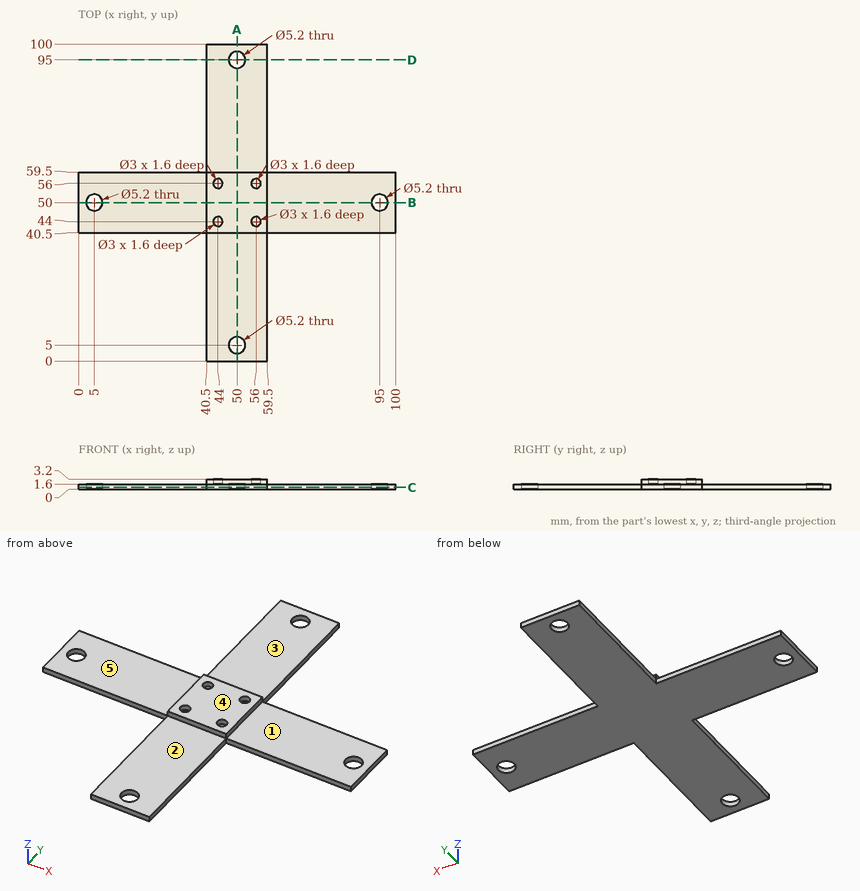
Geometry check sheet. Reference: drawing and pictorial views, mm from the part's lowest x, y, z. A direction names the side the tool comes from. Give positions to 0.01 mm unless a question says otherwise; leave off trailing zeros. Loops run counter-clockwise (first coordinate to the right, second up) from the corner with the lowest first, then second, coordinate; pieces in that order, holes last. Notation, with made-up numbers: (28, 31) -> (65, 31) arc R16 ccw to (65, 46) -> close; hole circle Ø6 at (80.5, 74). An arc over 180 degrees is marked (long way). Answer in a Markdown table with one row per item. Add a question column.
1) Set-up check for the marked faces 1, 2, 3, 4 and 5: record each of +Z, -Z, +X, -X, +Y, -Y from which the full face is reachable in a straight line by a thin tool's end or side.
2) Cross-section at A-A on x = 50. Record the boundary of the cut face in (y, z).
3) Cross-section at C-C on z = 0.55. Record the boundary of the cut face in (x, y), and give its area (3 significant figures).
4) Cross-section at D-D on y = 95. Record the boundary of the cut face in (x, z), and give its area (3 significant figures).
5) Material ranges on probe 1 along Y at (x, z) = (44, 2.1); probe 2 along Y at (x, z) = (50, 1.25); probe 3 along Z at (x, y) = (9.5, 44), recorded low to high. Write a range as from..to.
6) Gauge pin test, flat ends, axial feed: P1, Ø0.5, axis at y = 47, z = 2.5, coming from the -X side; P2, Ø0.5, axis at x = 79.5, z = 1, coming from the -Y side; P3, Ø0.9, axis at x = 44.5, y = 56.5, coming from the +Z side. Record the tip position at first contact, or that the pin passes through.
Outcome:
| question | item | result |
|---|---|---|
| 1 | face 1 | +Z, +X, +Y, -Y |
| 1 | face 2 | +Z, +X, -X, -Y |
| 1 | face 3 | +Z, +X, -X, +Y |
| 1 | face 4 | +Z, +X, -X, +Y, -Y |
| 1 | face 5 | +Z, -X, +Y, -Y |
| 2 | outline | (0, 0) -> (2.4, 0) -> (2.4, 1.6) -> (0, 1.6) -> close; (7.6, 0) -> (92.4, 0) -> (92.4, 1.6) -> (59.5, 1.6) -> (59.5, 3.2) -> (40.5, 3.2) -> (40.5, 1.6) -> (7.6, 1.6) -> close; (97.6, 0) -> (100, 0) -> (100, 1.6) -> (97.6, 1.6) -> close |
| 3 | outline | (0, 40.5) -> (40.5, 40.5) -> (40.5, 0) -> (59.5, 0) -> (59.5, 40.5) -> (100, 40.5) -> (100, 59.5) -> (59.5, 59.5) -> (59.5, 100) -> (40.5, 100) -> (40.5, 59.5) -> (0, 59.5) -> close; hole circle Ø5.2 at (5, 50); hole circle Ø5.2 at (50, 5); hole circle Ø5.2 at (50, 95); hole circle Ø5.2 at (95, 50) |
| 3 | area | 3,350 mm^2 |
| 4 | outline | (40.5, 0) -> (47.4, 0) -> (47.4, 1.6) -> (40.5, 1.6) -> close; (52.6, 0) -> (59.5, 0) -> (59.5, 1.6) -> (52.6, 1.6) -> close |
| 4 | area | 22.1 mm^2 |
| 5 | probe 1 | y = 40.5..42.5, 45.5..54.5, 57.5..59.5 |
| 5 | probe 2 | y = 0..2.4, 7.6..92.4, 97.6..100 |
| 5 | probe 3 | z = 0..1.6 |
| 6 | P1 | stops at x = 40.5 |
| 6 | P2 | stops at y = 40.5 |
| 6 | P3 | stops at z = 1.6 |
